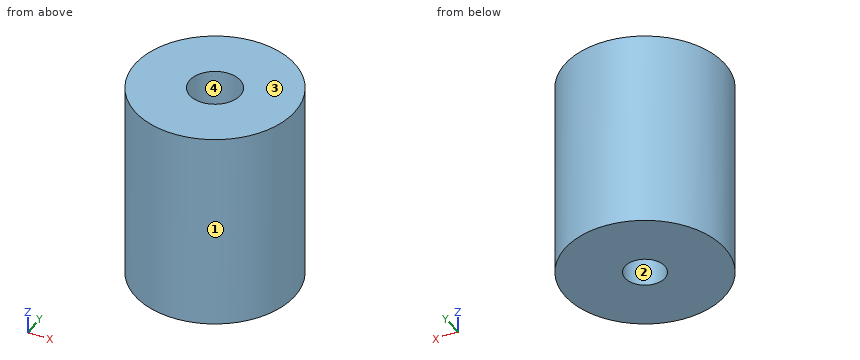
```python
from build123d import *

# Parameters (mm, degrees)
SKETCH1_R           = 10
BOSS_EXTRUDE1_DEPTH = 25
SKETCH2_R           = 3.175
CUT_EXTRUDE1_DEPTH  = 12.5
SKETCH3_R           = 2.5
CUT_EXTRUDE2_DEPTH  = 29.722813233


with BuildPart() as part:
    # Sketch1 → Boss-Extrude1 (new body)
    with BuildSketch(Plane.XY.offset(25)):
        with Locations(Location((0, 0, 0), (0, 0, 180))):
            Circle(SKETCH1_R)
    extrude(amount=-BOSS_EXTRUDE1_DEPTH)

    # Sketch2 → Cut-Extrude1 (cut)
    with BuildSketch(Plane.XY.offset(25)):
        with Locations(Location((0, 0, 0), (0, 0, 180))):
            Circle(SKETCH2_R)
    extrude(amount=-CUT_EXTRUDE1_DEPTH, mode=Mode.SUBTRACT)

    # Sketch3 → Cut-Extrude2 (cut, through all)
    with BuildSketch(Plane(origin=(0, 0, 0), x_dir=(-1, 0, 0), z_dir=(0, 0, -1))):
        Circle(SKETCH3_R)
    extrude(amount=-CUT_EXTRUDE2_DEPTH, mode=Mode.SUBTRACT)


solid = part.part
```
Model file for the job. Use its own axes, mm. Face numbers are marked on the shaded views. Round coordinates to 2 decimals unless told otherwise and drop trailing zeros. Write each loop counter-clockwise with the first axis right and the second up, starting at its lowest first coordinate (ties: lowest second). Pieces come first, ordered by that corner, then holes. Notation, with made-up numbers: (84, -11) - (100, -11) arc R26 ccw to (100, 3) - close; hole circle Ø6 at (79, 56). An arc over 180 degrees is marked (long way). One line per item, written item: value.
(1) Cut at C-C, the plane z = 13.5. Give the cut face in (x, y) (3 decimals), plus the area to 3 significant figures.
Values follow:
outline: circle Ø20 at (0, 0); hole circle Ø6.35 at (0, 0)
area: 282 mm²
(2) Cut at B-B, the plane x = 1.25. Give the cut face in (y, z).
Values follow:
outline: (-9.92, 0) - (-2.17, 0) - (-2.17, 12.5) - (-2.92, 12.5) - (-2.92, 25) - (-9.92, 25) - close; (2.17, 0) - (9.92, 0) - (9.92, 25) - (2.92, 25) - (2.92, 12.5) - (2.17, 12.5) - close
(3) Two-plate mould, pull along X, no slides. Class the marked faces 1, 2, 3 and 4: pulls with the +X half, pulls with the -X half, needs draft (parallel to the pull), parting line crosses it, or undercut.
Values follow:
face 1: parting line crosses it
face 2: undercut
face 3: needs draft
face 4: undercut
(4) Wall check: probe 1 along Y at (x, z) = (0, 22.5) (3 decimals); probe 2 along Y at (x, z) = (-0.5, 21); probe 3 along Z at (x, y) = (-1, 2.5). Give the ranges that are in metal, low to high.
Values follow:
probe 1: y = -10 to -3.175, 3.175 to 10
probe 2: y = -9.99 to -3.14, 3.14 to 9.99
probe 3: z = 0 to 12.5
(5) Cut at A-A, the plane y = 0. Give the cut face in (x, z) (3 decimals), plus the area to 3 significant figures.
Values follow:
outline: (-10, 0) - (-2.5, 0) - (-2.5, 12.5) - (-3.175, 12.5) - (-3.175, 25) - (-10, 25) - close; (2.5, 0) - (10, 0) - (10, 25) - (3.175, 25) - (3.175, 12.5) - (2.5, 12.5) - close
area: 358 mm²
(6) Drop flat-ended pins along their axis: P1, Ø8, axis at x = -7.5, z = 14, coming from the -Y side; P2, Ø4, axis at x = -4, z = 16, coming from the +Y side; P3, Ø1.9, axis at x = 0.5, y = 0, coming from the +Z side; P4, Ø2, axis at x = -7.5, z = 7.5, coming from the -Y side. Give the stop position or say it passes through.
Values follow:
P1: stops at y = -9.37
P2: stops at y = 9.8
P3: passes through
P4: stops at y = -7.6
(7) Cut at D-D, the plane y = 3.5. Give the cut face in (x, z).
Values follow:
outline: (-9.37, 0) - (9.37, 0) - (9.37, 25) - (-9.37, 25) - close
